Geometry check sheet. Reference: the model listing, model coordinates, mm. Give positions to 0.01 mm unless a question says otherwise; leave off trailing zeros. Write each loop counter-clockwise with the first axis right and the second up, starting at its lowest first coordinate (ties: lowest second). Pieces come first, ordered by that corner, then holes. Notation, with made-up numbers: (83.25, 37.25) - (120.25, 37.25) arc R20 ccw to (120.25, 71.25) - close; hole circle Ø2 at (72.5, 85). An arc over 180 degrees is marked (long way). Use a Markdown table: item, result.
```python
from build123d import *

# Parameters (mm, degrees)
SKETCH1_W                = 350
SKETCH1_H                = 400
BOSS_EXTRUDE1_DEPTH      = 15
BOSS_EXTRUDE2_DEPTH      = 10
BOSS_EXTRUDE2_DEPTH_BACK = 10
SKETCH3_R                = 12.5
SKETCH3_R_2              = 10
BOSS_EXTRUDE3_DEPTH      = 10
BOSS_EXTRUDE3_DEPTH_BACK = 10
SKETCH4_R                = 12.5
SKETCH4_R_2              = 10
CUT_EXTRUDE1_DEPTH       = 74
SKETCH6_R                = 7.5
BOSS_EXTRUDE4_DEPTH      = 10
BOSS_EXTRUDE5_DEPTH      = 5


with BuildPart() as part:
    # Sketch1 → Boss-Extrude1 (new body)
    with BuildSketch(Plane.XY):
        Rectangle(SKETCH1_W, SKETCH1_H)
    extrude(amount=BOSS_EXTRUDE1_DEPTH)

    # Sketch3 → Boss-Extrude2 (add, two sides: drawn at the far end of the back side and taken through both)
    # profile 1 of 2: a face of its own
    with BuildSketch(Plane(origin=(0, 100, 0), x_dir=(1, 0, 0), z_dir=(0, 1, 0)).offset(-BOSS_EXTRUDE2_DEPTH_BACK)):
        with BuildLine():
            ThreePointArc((-175, 12.5), (-178.661165235, 3.661165235), (-187.5, 0))
            Line((-187.5, 0), (-127.5, 0))
            Line((-127.5, 0), (-182.508319468, 23.960066556))
            ThreePointArc((-182.508319468, 23.960066556), (-177.04423588, 19.350328216), (-175, 12.5))
        make_face()
    # profile 2 of 2: a face of its own
    with BuildSketch(Plane(origin=(0, 100, 0), x_dir=(1, 0, 0), z_dir=(0, 1, 0)).offset(-BOSS_EXTRUDE2_DEPTH_BACK)):
        with Locations((-187.5, 12.5)):
            Circle(SKETCH3_R)
        with Locations(Location((-187.5, 12.5, 0), (0, 0, 270))):
            Circle(SKETCH3_R_2, mode=Mode.SUBTRACT)
    extrude(amount=BOSS_EXTRUDE2_DEPTH + BOSS_EXTRUDE2_DEPTH_BACK)

    # Sketch4 → Boss-Extrude3 (add, two sides: drawn at the far end of the back side and taken through both)
    # profile 1 of 2: a face of its own
    with BuildSketch(Plane(origin=(0, -100, 0), x_dir=(1, 0, 0), z_dir=(0, 1, 0)).offset(-BOSS_EXTRUDE3_DEPTH_BACK)):
        with Locations((-187.5, 12.5)):
            Circle(SKETCH4_R)
        with Locations(Location((-187.5, 12.5, 0), (0, 0, 270))):
            Circle(SKETCH4_R_2, mode=Mode.SUBTRACT)
    # profile 2 of 2: a face of its own
    with BuildSketch(Plane(origin=(0, -100, 0), x_dir=(1, 0, 0), z_dir=(0, 1, 0)).offset(-BOSS_EXTRUDE3_DEPTH_BACK)):
        with BuildLine():
            Line((-127.5, 0), (-182.508319468, 23.960066556))
            ThreePointArc((-182.508319468, 23.960066556), (-177.04423588, 19.350328216), (-175, 12.5))
            ThreePointArc((-175, 12.5), (-178.661165235, 3.661165235), (-187.5, 0))
            Line((-187.5, 0), (-127.5, 0))
        make_face()
    extrude(amount=BOSS_EXTRUDE3_DEPTH + BOSS_EXTRUDE3_DEPTH_BACK)

    # Sketch5 → Cut-Extrude1 (cut)
    with BuildSketch(Plane(origin=(0, 0, 0), x_dir=(-1, 0, 0), z_dir=(0, 0, -1))):
        with BuildLine():
            Line((-175, 200), (-175, 170))
            ThreePointArc((-175, 170), (-166.213203436, 191.213203436), (-145, 200))
            Line((-145, 200), (-175, 200))
        make_face()
        with BuildLine():
            ThreePointArc((-145, -200), (-166.213203436, -191.213203436), (-175, -170))
            Line((-175, -170), (-175, -200))
            Line((-175, -200), (-145, -200))
        make_face()
        with BuildLine():
            ThreePointArc((175, -170), (166.213203436, -191.213203436), (145, -200))
            Line((145, -200), (175, -200))
            Line((175, -200), (175, -170))
        make_face()
        with BuildLine():
            Line((175, 200), (145, 200))
            ThreePointArc((145, 200), (166.213203436, 191.213203436), (175, 170))
            Line((175, 170), (175, 200))
        make_face()
    extrude(amount=-CUT_EXTRUDE1_DEPTH, mode=Mode.SUBTRACT)

    # Sketch6 → Boss-Extrude4 (add)
    with BuildSketch(Plane(origin=(0, 0, 0), x_dir=(-1, 0, 0), z_dir=(0, 0, -1))):
        with Locations(Location((-145, 40, 0), (0, 0, 180))):
            Circle(SKETCH6_R)
        with Locations(Location((-145, -40, 0), (0, 0, 180))):
            Circle(SKETCH6_R)
    extrude(amount=BOSS_EXTRUDE4_DEPTH)

    # Sketch7 → Boss-Extrude5 (add)
    with BuildSketch(Plane(origin=(0, 0, -10), x_dir=(-1, 0, 0), z_dir=(0, 0, -1))):
        with BuildLine():
            Line((-150, 50), (-140, 50))
            ThreePointArc((-140, 50), (-136.464466094, 48.535533906), (-135, 45))
            Line((-135, 45), (-135, -45))
            ThreePointArc((-135, -45), (-136.464466094, -48.535533906), (-140, -50))
            Line((-140, -50), (-150, -50))
            ThreePointArc((-150, -50), (-153.535533906, -48.535533906), (-155, -45))
            Line((-155, -45), (-155, 45))
            ThreePointArc((-155, 45), (-153.535533906, 48.535533906), (-150, 50))
        make_face()
    extrude(amount=BOSS_EXTRUDE5_DEPTH)


solid = part.part
```
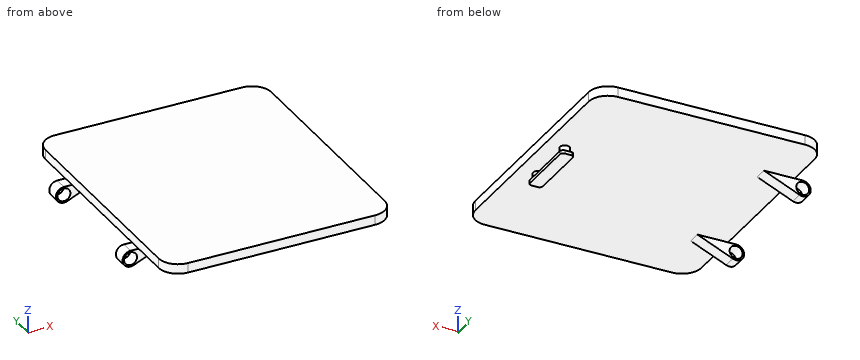
1) Depth check by flat-ended pin: P1, Ø12.5, axis at x = -170, z = -6.5, coming from the +Y side; P2, Ø8, axis at x = -161.5, y = 58.5, coming from the -Z side; P3, Ø12.5, axis at x = -146, z = -12.5, coming from the -Y side. Enter the tip coordinate at first touch or a pass-through.
Working result:
| item | result |
|---|---|
| P1 | stops at y = 110 |
| P2 | stops at z = 0 |
| P3 | stops at y = -110 |
2) Material ranges on L1, parallel to Z at x = -187, y = 100; L2, parallel to X at y = -168, z = 7; L3, parallel to Z at x = -2, y = -61, recorded low to high. Write a range as from..to.
Working result:
| item | result |
|---|---|
| L1 | z = -24.99..-22.49, -2.51..0 |
| L2 | x = -175..175 |
| L3 | z = 0..15 |
3) Section check C-C on y = 122.5. Record the boundary of the cut face in (x, z).
Working result:
| item | result |
|---|---|
| outline | (-175, 0) - (175, 0) - (175, 15) - (-175, 15) - close |
4) Section check A-A on y = -40. Record the boundary of the cut face in (x, z).
Working result:
| item | result |
|---|---|
| outline | (-175, 0) - (137.5, 0) - (137.5, -10) - (135, -10) - (135, -15) - (155, -15) - (155, -10) - (152.5, -10) - (152.5, 0) - (175, 0) - (175, 15) - (-175, 15) - close |
5) Section check B-B on x = 103. Record the boundary of the cut face in (y, z).
Working result:
| item | result |
|---|---|
| outline | (-200, 0) - (200, 0) - (200, 15) - (-200, 15) - close |
